Autodesk Inventor part; units mm, degrees
ref_plane "YZ Plane" through (0, 0, 0) normal (1, 0, 0) x (0, 1, 0)
ref_plane "XZ Plane" through (0, 0, 0) normal (0, 1, 0) x (-1, 0, 0)
ref_plane "XY Plane" through (0, 0, 0) normal (0, 0, 1) x (1, 0, 0)
sketch "Sketch1" plane through (0, 0, 0) normal (0, 1, 0) x (-1, 0, 0)
  line L0 (0, 0) -> (120, 0)
  line L1 (120, 0) -> (120, -130)
  line L2 (120, -130) -> (0, -130)
  line L3 (0, -130) -> (0, 0)
  line L4 (112.5, -12.5) -> (7.5, -12.5) construction
  line L5 (7.5, -12.5) -> (7.5, -117.5) construction
  line L6 (7.5, -117.5) -> (112.5, -117.5) construction
  line L7 (112.5, -117.5) -> (112.5, -12.5) construction
  circle A0 centre (112.5, -12.5) radius 1.524
  circle A1 centre (112.5, -117.5) radius 1.524
  circle A2 centre (7.5, -12.5) radius 1.524
  circle A3 centre (7.5, -117.5) radius 1.524
  line L8 (116.5, -130) -> (3.5, -130)
  line L9 (3.5, -130) -> (3.5, -144.7)
  line L10 (3.5, -144.7) -> (116.5, -144.7)
  line L11 (116.5, -144.7) -> (116.5, -130)
  line L12 (116.5, 0) -> (3.5, 0)
  line L13 (3.5, 0) -> (3.5, 9.25)
  line L14 (3.5, 9.25) -> (116.5, 9.25)
  line L15 (116.5, 9.25) -> (116.5, 0)
  point P0 (112.5, -65)
  point P1 (120, -65)
  point P2 (60, -117.5)
  point P3 (60, -130)
  point P4 (60, -144.7)
  point P5 (60, -130)
  point P6 (116.5, 4.625)
  point P7 (116.5, -137.35)
  point P8 (3.5, 0)
  point P9 (3.5, -130)
  dimension "d0" = 130
  dimension "d1" = 120
  dimension "d2" = 105
  dimension "d3" = 3.048
  dimension "d4" = 14.7
  dimension "d5" = 113
  dimension "d6" = 9.25
extrude "Extrusion1" add sketch "Sketch1" along normal blind 27.75
sketch "Sketch2" plane through (0, 27.75, 0) normal (0, 1, 0) x (1, 0, 0)
  circle A0 centre (-104.5, 137.35) radius 6.5
  circle A1 centre (-84.65, 137.35) radius 3.75
  circle A2 centre (-35.35, 137.35) radius 3.75
  line L0 (-116.5, 144.7) -> (-116.5, 130)
  line L1 (-3.5, 130) -> (-3.5, 144.7)
  point P0 (0, 0)
  point P1 (-116.5, 137.35)
  point P2 (-116.5, 137.35)
  point P3 (-116.5, 137.35)
  point P4 (-116.5, 137.35)
  point P5 (-3.5, 137.35)
  dimension "d9" = 13
  dimension "d10" = 7.5
  dimension "d11" = 12
  dimension "d12" = 31.85
  dimension "d13" = 31.85
extrude "Extrusion2" add sketch "Sketch2" along normal blind 16
properties part number "Radiator"
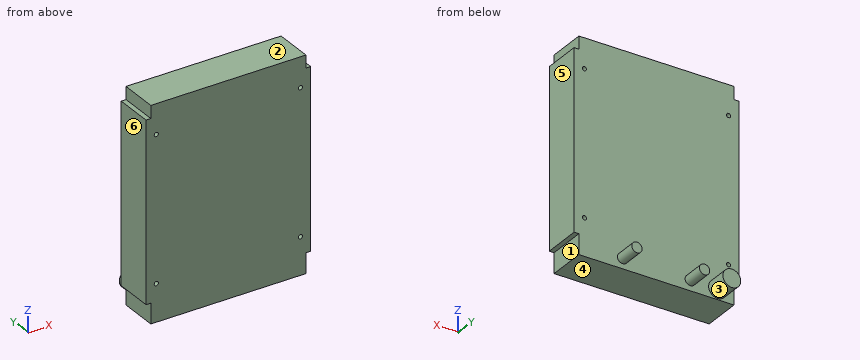
Input: part model. Units: mm. Frame: model coordinates. Face numbers are marked on the shaded views. A direction names the side the tool comes from. Give positions to 0.01 mm unless a question says otherwise; leave off trailing zeros. Write each loop counter-clockwise with the first axis right and the second up, starting at its lowest first coordinate (ties: lowest second). Pieces come first, ordered by that corner, then holes. Notation, with made-up numbers: (18, 23) - (77, 23) arc R19 cw to (77, 45) - close; hole circle Ø10 at (57.25, -29). An arc over 180 degrees is marked (long way). Write item = value, one per line. Start each with the question number.
1. Mould query, pull axis X, two halves, no side actions, for the marked faces 3, 4, 5 and 6. Classes: released by +X, released by -X, zero draft, split by the parting line, or undercut.
2. First-contact query: pin 1 Ø1.8 at (x, z) = (-112.5, -117.5) entering from +Y; pin 2 Ø16 at (y, z) = (11, -139.5) entering from -X; pin 3 Ø16 at (y, z) = (12, -139) entering from +X; pin 4 Ø6 at (x, z) = (-53, -26.5) entering from +Y. Flat tips, straight axial feed; report the tip coordinate or a pass-through.
3. Section query C-C, the plane x = -50.5. Output: boundary loops of the cut face in (y, z), then the cut area to 3 significant figures.
4. Section query A-A, the plane x = -104.5. Output: boundary loops of the cut face in (y, z), then the cut area to 3 significant figures.
5. Section query B-B, the plane z = -49.5. Output: boundary loops of the cut face in (x, y), then the cut area to 3 significant figures.
6. Ray query, L1, parallel to X at y = 8, z = -117.5; L2, parallel to Z at x = -112.5, y = 10; L3, parallel to Z at x = -7, y = 14. Return the intervals inside material, ascending.
7. Access query for the marked faces 1 and 2. Directions: +Z, -Z, +X, -X, +Y, -Y. A direction counts if a zero-diameter tool reaches every point of the face in a straight line with its end or side. Return the directions, or none.
Check sheet entries:
q1.face_3 = undercut
q1.face_4 = zero draft
q1.face_5 = released by +X
q1.face_6 = released by -X
q2.pin_1 = through
q2.pin_2 = -116.5
q2.pin_3 = -3.5
q2.pin_4 = 27.75
q3.outline = (0, -144.7) - (27.75, -144.7) - (27.75, 9.25) - (0, 9.25) - close
q3.area = 4,270 mm2
q4.outline = (0, -144.7) - (27.75, -144.7) - (27.75, -143.85) - (43.75, -143.85) - (43.75, -130.85) - (27.75, -130.85) - (27.75, 9.25) - (0, 9.25) - close
q4.area = 4,480 mm2
q5.outline = (-120, 0) - (0, 0) - (0, 27.75) - (-120, 27.75) - close
q5.area = 3,330 mm2
q6.L1 = -120 to -114.02, -110.98 to -9.02, -5.98 to 0
q6.L2 = -144.7 to -119.02, -115.98 to -14.02, -10.98 to 9.25
q6.L3 = -144.7 to -118.94, -116.06 to -13.94, -11.06 to 9.25
q7.face_1 = -Z, +X, +Y, -Y
q7.face_2 = +Z, +X, -X, +Y, -Y
